Geometry: final body of the model. Coordinates: model frame, mm. Face numbers are marked on the shaded views. A direction names the side the tool comes from. Give positions to 0.01 mm unless a question says otherwise; leave off trailing zeros. Loops run counter-clockwise (first coordinate to the right, second up) from the corner with the lowest first, then second, coordinate; pieces in that order, holes last.
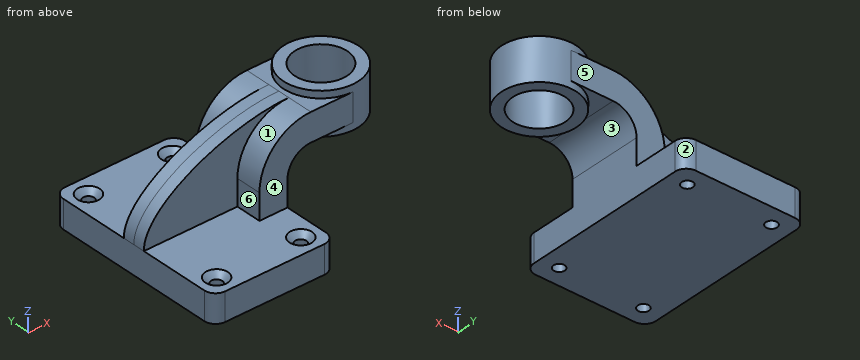
from build123d import *

# Parameters (mm, degrees)
F1_DEPTH       = 63.5
F0_W           = 25.4
F0_H           = 19.05
F2_DEPTH       = 25.4
F3_DEPTH       = 7.9375
F5_R           = 7.62
F7_D           = 7.62
F7_CSINK_D     = 15.24
F7_CSINK_ANGLE = 90
F8_D           = 7.62
F8_CSINK_D     = 15.24
F8_CSINK_ANGLE = 90
F10_D          = 35.56


with BuildPart() as f1:
    # F0 (on Front) → F1 (new body, symmetric)
    with BuildSketch(Plane.XZ):
        Polygon((22.225, 9.525), (-41.275, 9.525), (-41.275, -9.525), (41.275, -9.525), (41.275, 9.525), align=None)
    extrude(amount=F1_DEPTH, both=True)

    # F0 (on Front) → F2 (join, symmetric)
    with BuildSketch(Plane.XZ):
        with BuildLine():
            Line((22.225, 27.0002), (22.225, 9.525))
            Line((22.225, 9.525), (41.275, 9.525))
            Line((41.275, 9.525), (41.275, 27.0002))
            ThreePointArc((41.275, 27.0002), (45.9246798487, 38.2255201513), (57.15, 42.8752))
            Line((57.15, 42.8752), (60.325, 42.8752))
            Line((60.325, 42.8752), (60.325, 61.9252))
            Line((60.325, 61.9252), (57.15, 61.9252))
            ThreePointArc((57.15, 61.9252), (32.4542956671, 51.6959043329), (22.225, 27.0002))
        make_face()
        with Locations((73.025, 52.4002)):
            Rectangle(F0_W, F0_H)
    extrude(amount=F2_DEPTH, both=True)

    # F0 (on Front) → F3 (join, symmetric)
    with BuildSketch(Plane.XZ):
        with BuildLine():
            add(Edge.make_bspline(
                [(-41.275, 9.525), (-41.3618534803, 36.8419066072), (17.3745620996, 62.5231936574), (57.15, 61.9252)],
                knots=[0, 0, 0, 0, 111.5045361635, 111.5045361635, 111.5045361635, 111.5045361635], degree=3))
            Line((-41.275, 9.525), (22.225, 9.525))
            Line((22.225, 9.525), (22.225, 27.0002))
            ThreePointArc((22.225, 27.0002), (32.4542956671, 51.6959043329), (57.15, 61.9252))
        make_face()
    extrude(amount=F3_DEPTH, both=True)

    # F0 (on Front) → F4 (revolve)
    with BuildSketch(Plane.XZ):
        Polygon((85.725, 66.675), (85.725, 61.9252), (85.725, 42.8752), (85.725, 38.1), (111.125, 38.1), (111.125, 66.675), align=None)
    revolve(axis=Axis((85.725, 0, 52.3875), (0, 0, 1)))

    # F5
    f5_edges = [f1.edges().sort_by_distance(p)[0] for p in [
        (-41.275, -63.5, 0),
        (41.275, -63.5, 0),
        (-41.275, 63.5, 0),
        (41.275, 63.5, 0),
    ]]
    fillet(f5_edges, radius=F5_R)

    # F7 (through all)
    with Locations(Plane.XY.offset(9.525)):
        with Locations((-28.575, 50.8)):
            CounterSinkHole(F7_D / 2, F7_CSINK_D / 2, counter_sink_angle=F7_CSINK_ANGLE)

    # F8 (through all)
    with Locations(Plane.XY.offset(9.525)):
        with Locations((-28.575, -50.8), (28.575, -50.8), (28.575, 50.8)):
            CounterSinkHole(F8_D / 2, F8_CSINK_D / 2, counter_sink_angle=F8_CSINK_ANGLE)

    # F10 (through all)
    with Locations(Plane.XY.offset(66.675)):
        with Locations((85.725, 0)):
            Hole(F10_D / 2)


solid = f1.part
Item 1: Section query C-C on y = -15. Return loops of the section in (x, z) (3 decimals).
Values follow:
outline: (-41.275, -9.525) - (41.275, -9.525) - (41.275, 27) arc R15.875 cw to (57.15, 42.875) - (65.227, 42.875) - (65.227, 38.1) - (76.179, 38.1) - (76.179, 66.675) - (65.227, 66.675) - (65.227, 61.925) - (57.15, 61.925) arc R34.925 ccw to (22.225, 27) - (22.225, 9.525) - (-41.275, 9.525) - close; (95.271, 38.1) - (106.223, 38.1) - (106.223, 66.675) - (95.271, 66.675) - close
Item 2: Section query A-A on y = -50.8. Return loops of the section in (x, z) (3 decimals), plus the area to 3 significant figures.
Values follow:
outline: (-41.275, -9.525) - (-32.385, -9.525) - (-32.385, 5.715) - (-36.195, 9.525) - (-41.275, 9.525) - close; (-24.765, -9.525) - (24.765, -9.525) - (24.765, 5.715) - (20.955, 9.525) - (-20.955, 9.525) - (-24.765, 5.715) - close; (32.385, -9.525) - (41.275, -9.525) - (41.275, 9.525) - (36.195, 9.525) - (32.385, 5.715) - close
area: 1,250 mm2
Item 3: Pin query (flat end, axial travel): pin 1 (6 mm diameter, centred on x = -28.575, y = -50.8, fed in from -Z); pin 2 (14 mm diameter, centred on y = -15.5, z = 20.5, fed in from -X) (3 decimals); pin 3 (5 mm diameter, centred on y = 46.5, z = 4.5, fed in from +X) (3 decimals); pin 4 (3 mm diameter, centred on x = -15.5, z = 14, fed in from -Y). Return the tip coordinate at first contact, or that it passes through.
Values follow:
pin 1: passes through
pin 2: stops at x = 22.225
pin 3: stops at x = 41.275
pin 4: stops at y = -7.94
Item 4: Ray query, probe 1 along X at (y, z) = (-50.8, -2) (3 decimals); probe 2 along Z at (x, y) = (-4, -16.5) (3 decimals); probe 3 along X at (y, z) = (-15.5, 11) (3 decimals). Return the intervals inside material, ascending.
Values follow:
probe 1: x = -41.275 to -32.385, -24.765 to 24.765, 32.385 to 41.275
probe 2: z = -9.525 to 9.525
probe 3: x = 22.225 to 41.275
Item 5: Section query B-B on z = -4.5. Return loops of the section in (x, y) (3 decimals), plus the area to 3 significant figures.
Values follow:
outline: (-41.275, -55.88) arc R7.62 ccw to (-33.655, -63.5) - (33.655, -63.5) arc R7.62 ccw to (41.275, -55.88) - (41.275, 55.88) arc R7.62 ccw to (33.655, 63.5) - (-33.655, 63.5) arc R7.62 ccw to (-41.275, 55.88) - close; hole circle Ø7.62 at (-28.575, -50.8); hole circle Ø7.62 at (-28.575, 50.8); hole circle Ø7.62 at (28.575, -50.8); hole circle Ø7.62 at (28.575, 50.8)
area: 10,300 mm2
Item 6: Set-up query: the marked faces 4, 5 and 6. Return all of +Z, -Z, +X, -X, +Y, -Y with unobstructed straight access to the full face (end or side cutting, diameter ignored); none if empty.
Values follow:
face 4: +Z, +X, -X, -Y
face 5: +Z, +X, -X, +Y
face 6: +Z, -X, -Y
Item 7: Draft query along X for the marked faces 1, 2 and 3. Return one class per face: +X half, -X half, draft (parallel to the pull), parting line (faces both ways), or undercut.
Values follow:
face 1: -X half
face 2: +X half
face 3: undercut
